Part model, mm, in its own coordinate system. A direction names the side the tool comes from. Give positions to 0.01 mm unless a question says otherwise; leave off trailing zeros. Order: outer loops, then holes, each group sorted by start corner. A loop starts at its lowest first (then second) coordinate and runs counter-clockwise, first axis right, second up.
from build123d import *

# Parameters (mm, degrees)
BOSS_EXTRUDE1_DEPTH = 200
SKETCH2_W           = 165
SKETCH2_H           = 550
CUT_EXTRUDE1_DEPTH  = 170
CUT_EXTRUDE2_DEPTH  = 50
CUT_EXTRUDE5_DEPTH  = 110
SCALE1_SCALE        = 0.1
SKETCH7_W           = 4
SKETCH7_H           = 9
CUT_EXTRUDE6_DEPTH  = 17.5


with BuildPart() as part:
    # Sketch1 → Boss-Extrude1 (new body)
    with BuildSketch(Plane.XY):
        Polygon((0, 404.145188433), (-350, 202.072594216), (-350, -202.072594216), (0, -404.145188433), (350, -202.072594216), (350, 202.072594216), align=None)
    extrude(amount=BOSS_EXTRUDE1_DEPTH)

    # Sketch2 → Cut-Extrude1 (cut)
    with BuildSketch(Plane.XY.offset(200)):
        with Locations((-92.5, 0)):
            Rectangle(SKETCH2_W, SKETCH2_H)
        with Locations((92.5, 0)):
            Rectangle(SKETCH2_W, SKETCH2_H)
    extrude(amount=-CUT_EXTRUDE1_DEPTH, mode=Mode.SUBTRACT)

    # Sketch4 → Cut-Extrude2 (cut)
    with BuildSketch(Plane(origin=(0, 0, 0), x_dir=(-1, 0, 0), z_dir=(0, 0, -1))):
        with BuildLine():
            Line((-85, 20.592361582), (85, 20.592361582))
            ThreePointArc((85, 20.592361582), (105.592361582, 0), (85, -20.592361582))
            Line((85, -20.592361582), (-85, -20.592361582))
            ThreePointArc((-85, -20.592361582), (-105.592361582, 0), (-85, 20.592361582))
        make_face()
    extrude(amount=-CUT_EXTRUDE2_DEPTH, mode=Mode.SUBTRACT)

    # Sketch6 → Cut-Extrude5 (cut)
    with BuildSketch(Plane.XY.offset(200)):
        Polygon((-10, 275), (-10, 284.635017666), (10, 284.635017666), (10, 275), (63.624515443, 275), (63.624515443, 315), (-63.624515443, 315), (-63.624515443, 275), align=None)
        Polygon((-10, -275), (-63.624515443, -275), (-63.624515443, -315), (63.624515443, -315), (63.624515443, -275), (10, -275), (10, -284.635017666), (-10, -284.635017666), align=None)
    extrude(amount=-CUT_EXTRUDE5_DEPTH, mode=Mode.SUBTRACT)


with BuildPart() as part_1:
    # Scale1: scaled about (0, 0, 90.714754865)
    add(part.part.scale(SCALE1_SCALE).moved(Location((0, 0, 81.643279379))))

    # Sketch7 → Cut-Extrude6 (cut)
    with BuildSketch(Plane.ZY.offset(35)):
        with Locations((99.650437811, 10.707259422)):
            Rectangle(SKETCH7_W, SKETCH7_H)
    extrude(amount=-CUT_EXTRUDE6_DEPTH, mode=Mode.SUBTRACT)


solid = part_1.part
Item 1: Band-saw the part on C-C on y = -13.5. List the corners of the cut face in (x, z).
Item 2: Drill centre lines: probe 1 along X at (y, z) = (-15, 87.75); probe 2 along X at (y, z) = (21, 98); probe 3 along Y at (x, z) = (4, 92). Where is each one in solid material? Low to high.
Item 3: Band-saw the part on B-B on z = 89.5. List the corners of the cut face in (x, y).
Item 4: Band-saw the part on D-D on x = -2. List the corners of the cut face in (y, z).
Item 5: Pull direction X, two halves, no side cores. Call faces 1 (the face through (-17.5, 0, 93)), 2 (the face through (17.745, 30.169, 91.503)), 3 (the face through (-26, 6.207, 100)): released by +X, released by -X, zero draft, split by the parting line, or undercut.
Item 6: Band-saw the part on A-A on y = 0. List the corners of the cut face in (x, z), plus the area to 3 significant figures.
Item 7: Which spindle directions (+Z, -Z, +X, -X, +Y, -Y) get a long thin tool onto all of the face, cutting with end or side? Do faces 4 (the face through (0, -28.464, 96)), 5 (the face through (0, -2.059, 83)), 6 (the face through (-26, 15.207, 100)), 7 (the face through (-10.56, 0.05, 83.12)). Say none if no direction does.
Item 8: Drop flat-ended pins along their axis: P1, Ø7, axis at x = -29, y = 10.5, coming from the +Z side; P2, Ø5, axis at x = -9, z = 95, coming from the -Y side; P3, Ø5, axis at y = 29, z = 97.5, coming from the +X side; P4, Ø18, axis at x = -7.5, y = -3, coming from the +Z side. Give the stop position or say it passes through.
Working result:
1. outline: (-35, 81.64) - (35, 81.64) - (35, 101.64) - (17.5, 101.64) - (17.5, 84.64) - (1, 84.64) - (1, 101.64) - (-1, 101.64) - (-1, 84.64) - (-17.5, 84.64) - (-17.5, 101.64) - (-35, 101.64) - close
2. probe 1: x = -35 to -17.5, -1 to 1, 17.5 to 35
2. probe 2: x = -33.63 to -17.5, -1 to 1, 17.5 to 33.63
2. probe 3: y = -38.11 to -31.5, 31.5 to 38.11
3. outline: (-35, -20.21) - (0, -40.41) - (35, -20.21) - (35, 20.21) - (0, 40.41) - (-35, 20.21) - close; hole (-17.5, -27.5) - (-1, -27.5) - (-1, 27.5) - (-17.5, 27.5) - close; hole (1, -27.5) - (17.5, -27.5) - (17.5, 27.5) - (1, 27.5) - close
4. outline: (-39.26, 81.64) - (-2.06, 81.64) - (-2.06, 84.64) - (-27.5, 84.64) - (-27.5, 90.64) - (-31.5, 90.64) - (-31.5, 101.64) - (-39.26, 101.64) - close; (2.06, 81.64) - (39.26, 81.64) - (39.26, 101.64) - (31.5, 101.64) - (31.5, 90.64) - (27.5, 90.64) - (27.5, 84.64) - (2.06, 84.64) - close
5. face 1: undercut
5. face 2: released by +X
5. face 3: zero draft
6. outline: (-35, 81.64) - (-10.56, 81.64) - (-10.56, 84.64) - (-17.5, 84.64) - (-17.5, 101.64) - (-35, 101.64) - close; (-1, 86.64) - (1, 86.64) - (1, 101.64) - (-1, 101.64) - close; (10.56, 81.64) - (35, 81.64) - (35, 101.64) - (17.5, 101.64) - (17.5, 84.64) - (10.56, 84.64) - close
6. area: 772 mm2
7. face 4: +Z
7. face 5: -Z
7. face 6: +Z, -X
7. face 7: +Z, -Z
8. P1: stops at z = 97.65
8. P2: stops at y = -36.66
8. P3: stops at x = 24.1
8. P4: stops at z = 101.64
